Design review of the part built by this model. Coordinates are the model's own, in mm. A direction names the side the tool comes from. Give positions to 0.01 mm unless a question says otherwise; leave off trailing zeros. Order: outer loops, then holes, each group sorted by start corner. A loop starts at its lowest first (then second) coordinate and runs counter-clockwise, first axis right, second up.
Autodesk Inventor part; units mm, degrees
ref_plane "Work Plane1" through (0, 800, 0) normal (0, 1, 0) x (1, 0, 0)
ref_plane "YZ Plane" through (0, 0, 0) normal (1, 0, 0) x (0, 1, 0)
ref_plane "XZ Plane" through (0, 0, 0) normal (0, 1, 0) x (-1, 0, 0)
sketch "Sketch1" plane through (0, 0, 0) normal (0, 1, 0) x (-1, 0, 0)
  circle A0 centre (0, 0) radius 65
  dimension "d0" = 130
extrude "Beam" add sketch "Sketch1" along normal blind 800
ref_plane "Work Plane1" through (0, 800, 0) normal (0, 1, 0) x (1, 0, 0)
sketch "Sketch2" plane through (0, 800, 0) normal (0, 1, 0) x (1, 0, 0)
  line L0 (-68, 68) -> (68, 68)
  line L1 (68, 68) -> (68, -68)
  line L2 (68, -68) -> (-68, -68)
  line L3 (-68, -68) -> (-68, 68)
  line L4 (-68, 68) -> (68, -68) construction
  line L5 (68, 68) -> (-68, -68) construction
  point P0 (0, 0)
extrude "Connector" add sketch "Sketch2" along normal blind 10
sketch "Sketch6" plane through (0, 810, 0) normal (0, 1, 0) x (1, 0, 0)
  circle A0 centre (0, 0) radius 20
extrude "CableHole" cut sketch "Sketch6" against normal up to next
sketch "Sketch8" plane through (0, 800, 0) normal (0, -1, 0) x (1, 0, 0)
  point P0 (0, 0)
  point P1 (58, -58)
  point P2 (-58, -58)
  point P3 (-58, 58)
  point P4 (58, 58)
hole "Hole2" at (58, 800, -58) at (-58, 800, -58) at (-58, 800, 58) at (58, 800, 58) direction (0, 1, 0) diameter 6 depth 10 tip angle 118 counterbore diameter 9 counterbore depth 2
properties part number "RaAxis"
1. Take a section at D-D (y = 664.5). State the section outline as (x, z) points, then the cut area to 3 significant figures.
Recorded:
outline: circle Ø130 at (0, 0); hole circle Ø40 at (0, 0)
area: 12,000 mm2
2. Machinability: for faces 1 (the face through (-16, 810, -16)), 2 (the face through (-62, 394.4, -19.52)), which of the approach directions +Z, -Z, +X, -X, +Y, -Y give a long, thin tool a straight path to every point of the face, cutting with its end or side? Answer none if there is none.
Recorded:
face 1: +Z, -Z, +X, -X, +Y
face 2: -Y
3. Take a section at A-A (x = 0). State the section outline as (y, z) points.
Recorded:
outline: (0, -65) - (800, -65) - (800, -68) - (810, -68) - (810, -20) - (0, -20) - close; (0, 20) - (810, 20) - (810, 68) - (800, 68) - (800, 65) - (0, 65) - close
4. Take a section at B-B (z = 0). State the section outline as (x, y) points, then the cut area to 3 significant figures.
Recorded:
outline: (-68, 800) - (-65, 800) - (-65, 0) - (-20, 0) - (-20, 810) - (-68, 810) - close; (20, 0) - (65, 0) - (65, 800) - (68, 800) - (68, 810) - (20, 810) - close
area: 73,000 mm2
5. For pin 1 (10 mm diameter, centred on x = -59.5, z = 59, fed in from -Y); pin 2 (8 mm diameter, centred on x = 58, z = 58, fed in from -Y); pin 3 (7 mm diameter, centred on x = -58, z = -58, fed in from +Y); pin 4 (5 mm diameter, centred on y = 251, z = 0.5, fed in from +X), all flat-tipped, find the tip position at first contact; note any pin that passes through.
Recorded:
pin 1: stops at y = 800
pin 2: stops at y = 802
pin 3: stops at y = 810
pin 4: stops at x = 65
6. For line 1 along Z through (x, y) = (58, 801.3); line 2 along Z through (x, y) = (-58, 807), list the stretches that pass through material, from the lowest coordinate up.
Recorded:
line 1: z = -68 to -62.5, -53.5 to 53.5, 62.5 to 68
line 2: z = -68 to -61, -55 to 55, 61 to 68
7. Take a section at C-C (x = 34.5). State the section outline as (y, z) points.
Recorded:
outline: (0, -55.09) - (800, -55.09) - (800, -68) - (810, -68) - (810, 68) - (800, 68) - (800, 55.09) - (0, 55.09) - close
